The listing builds one solid part. Answer for the finished solid, in the listing's coordinates (mm). Face numbers are marked on the shaded views. A direction names the side the tool comes from. Give positions to 0.01 mm unless a question says otherwise; leave off trailing zeros. Write each loop counter-clockwise with the first axis right and the second up, starting at its lowest first coordinate (ties: lowest second). Pieces come first, ordered by that corner, then holes. Notation, with made-up numbers: (34.5, 69) -> (68.5, 69) arc R21 cw to (68.5, 89) -> close; hole circle Ø5 at (85.5, 31.25). An arc over 180 degrees is marked (long way). Use CSV: the item, a comma, the result in double quotes. Start each with the question number.
from build123d import *

# Parameters (mm, degrees)
F0_R     = 35.75
F0_R_2   = 10
F1_DEPTH = 2
F2_R     = 27
F2_R_2   = 10
F3_DEPTH = 10
F4_R     = 2


with BuildPart() as f1:
    # F0 (on Front) → F1 (new body)
    with BuildSketch(Plane.XZ):
        Circle(F0_R)
        Circle(F0_R_2, mode=Mode.SUBTRACT)
    extrude(amount=F1_DEPTH)

    # F2 (on face) → F3 (join)
    with BuildSketch(Plane(origin=(0, 0, 0), x_dir=(-1, 0, 0), z_dir=(0, 1, 0))):
        Circle(F2_R)
        Circle(F2_R_2, mode=Mode.SUBTRACT)
    extrude(amount=F3_DEPTH)

    # F4
    f4_edges = [f1.edges().sort_by_distance(p)[0] for p in [
        (27, 10, 0),
    ]]
    fillet(f4_edges, radius=F4_R)


solid = f1.part
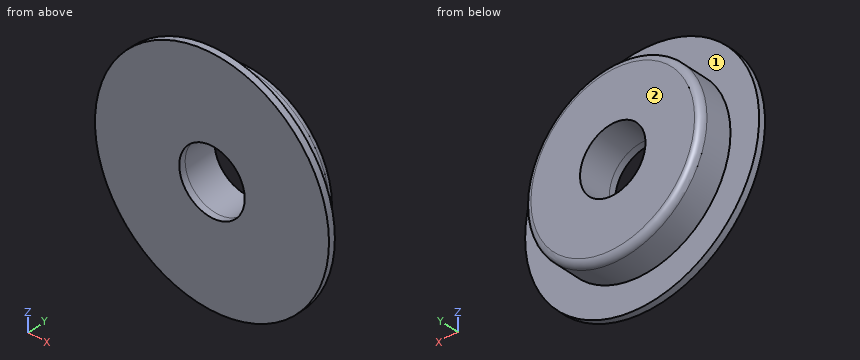
Q1. For the marked faces 1 and 2, determine the directions among +Z, -Z, +X, -X, +Y, -Y from which every point of the face is accessible in a straight line to the end or side of a thin tool.
Q2. Section B-B on z = 0 is taken. Give the vertices of the cut face in (x, y), then the cut area to 3 significant figures.
Q3. Flat-ended cylindrical pins translate along their axes: pin 1 Ø4 at (x, z) = (24, -24.5) entering from +Y; pin 2 Ø16 at (x, z) = (0, 0) entering from -Y; pin 3 Ø23 at (x, z) = (0, 0) entering from -Y; pin 4 Ø4 at (x, y) = (14, 3.5) entering from +Z. Find the tip coordinate at first contact, or state that the pin passes through.
Q4. Section C-C on y = 4 is taken. Give the vertices of the cut face in (x, z).
Q5. Section A-A on x = 0 is taken. Give the vertices of the cut face in (y, z), then the cut area to 3 significant figures.
Q6. Straight lines are drawn through the part: L1, parallel to Z at x = 0, y = 6.5; L2, parallel to Y at x = -18, z = 22; L3, parallel to X at y = 7.25, z = -5. For each, find the intervals that lie inside material, in ascending order.
Output:
1,face 1,"+Y"
1,face 2,"+Z, -Z, +X, -X, +Y"
2,outline,"(-35.75, -2) -> (-10, -2) -> (-10, 10) -> (-25, 10) arc R2 ccw to (-27, 8) -> (-27, 0) -> (-35.75, 0) -> close; (10, -2) -> (35.75, -2) -> (35.75, 0) -> (27, 0) -> (27, 8) arc R2 ccw to (25, 10) -> (10, 10) -> close"
2,area,"441 mm²"
3,pin 1,"y = 0"
3,pin 2,"through"
3,pin 3,"y = -2"
3,pin 4,"z = 24.19"
4,outline,"circle Ø54 at (0, 0); hole circle Ø20 at (0, 0)"
5,outline,"(-2, -35.75) -> (0, -35.75) -> (0, -27) -> (8, -27) arc R2 ccw to (10, -25) -> (10, -10) -> (-2, -10) -> close; (-2, 10) -> (10, 10) -> (10, 25) arc R2 ccw to (8, 27) -> (0, 27) -> (0, 35.75) -> (-2, 35.75) -> close"
5,area,"441 mm²"
6,L1,"-27 to -10, 10 to 27"
6,L2,"-2 to 0"
6,L3,"-26.53 to -8.66, 8.66 to 26.53"
